from build123d import *

# Parameters (mm, degrees)
EXTRUDE_1_DEPTH     = 18
SKETCH_4_R          = 2.1
CUT_EXTRUDE_3_DEPTH = 38
SKETCH_5_R          = 2.1
CUT_EXTRUDE_4_DEPTH = 38


with BuildPart() as part:
    # 草图1 → 凸台-拉伸1 (new body)
    with BuildSketch(Plane.XY):
        Polygon((0, 25), (0, 0), (25, 0), (25, 4), (4, 4), (4, 25), align=None)
    extrude(amount=EXTRUDE_1_DEPTH)

    # 草图4 → 切除-拉伸3 (cut)
    with BuildSketch(Plane(origin=(0, 4, 0), x_dir=(1, 0, 0), z_dir=(0, 1, 0))):
        with Locations(Location((13, -5, 0), (0, 0, 180))):
            Circle(SKETCH_4_R)
        with Locations(Location((13, -13, 0), (0, 0, 180))):
            Circle(SKETCH_4_R)
    extrude(amount=-CUT_EXTRUDE_3_DEPTH, mode=Mode.SUBTRACT)

    # 草图5 → 切除-拉伸4 (cut)
    with BuildSketch(Plane.ZY):
        with Locations(Location((5, 18, 0), (0, 0, 270))):
            Circle(SKETCH_5_R)
        with Locations(Location((13, 18, 0), (0, 0, 270))):
            Circle(SKETCH_5_R)
    extrude(amount=-CUT_EXTRUDE_4_DEPTH, mode=Mode.SUBTRACT)


solid = part.part
For this review, take the finished solid that the model builds, in its own axes (mm). A direction names the side the tool comes from. Give positions to 0.01 mm unless a question says otherwise; leave off trailing zeros. Order: outer loops, then holes, each group sorted by start corner. A loop starts at its lowest first (then second) coordinate and runs counter-clockwise, first axis right, second up. Notation, with made-up numbers: (17.5, 38.25) - (49.5, 38.25) arc R24 ccw to (49.5, 63.25) - close; hole circle Ø2 at (-8.5, 74). An arc over 180 degrees is marked (long way). Answer as a JSON object with one key per item and string values. Group by question number.
Item 1: Wall thickness on line 1 along Z through (x, y) = (3, 18); line 2 along Y through (x, z) = (23.5, 10.25): over which ranges is each line inside the solid? List them lowest first.
Item 2: Take a section at A-A on y = 18. Give the boundary of the cut face in (x, z).
Item 3: Take a section at D-D on y = 2.5. Give the boundary of the cut face in (x, z).
Item 4: Draft analysis for pull direction Z (two halves, no side actions). For faces 1 (the cylindrical face through (15.1, 2.03, 13.09)), 2 (the flat face through (3, 8, 0)), 3 (the flat face through (15, 4, 9)), state which applies: pulls with the +Z half, pulls with the -Z half, needs draft (parallel to the pull), parting line crosses it, or undercut.
Item 5: Machinability: for faces 4 (the flat face through (3, 8, 18)), 5 (the flat face through (4, 14, 9)), which of the approach directions +Z, -Z, +X, -X, +Y, -Y give a long, thin tool a straight path to every point of the face, cutting with its end or side? Answer none if there is none.
Item 6: Clearance check with flat-ended pins moving along their axes: pin 1 Ø6.5 at (y, z) = (18, 5) entering from +X; pin 2 Ø2 at (x, y) = (5.5, 11.5) entering from +Z; pin 3 Ø5.5 at (x, z) = (9.5, 11) entering from +Y. State where each tip first meets the part, or that it passes through.
Item 7: Take a section at B-B on z = 5. Give the boundary of the cut face in (x, y).
Reported:
{
 "1": {"line 1": "0 to 2.9, 7.1 to 10.9, 15.1 to 18", "line 2": "0 to 4"},
 "2": {"outline": "(0, 0) - (4, 0) - (4, 2.9) - (0, 2.9) - close; (0, 7.1) - (4, 7.1) - (4, 10.9) - (0, 10.9) - close; (0, 15.1) - (4, 15.1) - (4, 18) - (0, 18) - close"},
 "3": {"outline": "(0, 0) - (25, 0) - (25, 18) - (0, 18) - close; hole circle Ø4.2 at (13, 5); hole circle Ø4.2 at (13, 13)"},
 "4": {"face 1": "undercut", "face 2": "pulls with the -Z half", "face 3": "needs draft"},
 "5": {"face 4": "+Z, +X, -X, +Y, -Y", "face 5": "+Z, -Z, +X, +Y"},
 "6": {"pin 1": "x = 4", "pin 2": "through", "pin 3": "y = 4"},
 "7": {"outline": "(0, 0) - (10.9, 0) - (10.9, 4) - (4, 4) - (4, 15.9) - (0, 15.9) - close; (0, 20.1) - (4, 20.1) - (4, 25) - (0, 25) - close; (15.1, 0) - (25, 0) - (25, 4) - (15.1, 4) - close"}
}
